Can you work these out from the model? Positions are in its coordinate system, mm. A direction names the side the tool comes from. Give positions to 0.01 mm unless a question says otherwise; leave off trailing zeros. Loops run counter-clockwise (first coordinate to the right, second up) from the corner with the lowest first, then second, coordinate; pieces in that order, holes last. Notation, with made-up numbers: (36, 62) -> (78, 62) arc R12 cw to (78, 71) -> close; hole circle Ø1 at (-9, 11). An arc over 180 degrees is marked (long way). Use CSV: the item, a comma, the result in double quotes.
Autodesk Inventor part; units mm, degrees
ref_plane "YZ Plane" through (0, 0, 0) normal (1, 0, 0) x (0, 1, 0)
ref_plane "XZ Plane" through (0, 0, 0) normal (0, 1, 0) x (-1, 0, 0)
ref_plane "XY Plane" through (0, 0, 0) normal (0, 0, 1) x (1, 0, 0)
sketch "Эскиз1" plane through (0, 0, 0) normal (0, 1, 0) x (-1, 0, 0)
  line L0 (0, 0) -> (8, 0) construction
  line L1 (8, 0) -> (8, 4)
  line L2 (8, 4) -> (13, 4)
  line L3 (13, 4) -> (13, 27)
  line L4 (13, 27) -> (20, 27)
  line L5 (0, 0) -> (0, 86)
  line L6 (0, 0) -> (-8, 0) construction
  line L7 (-8, 0) -> (-8, 4)
  line L8 (-8, 4) -> (-13, 4)
  line L9 (-13, 4) -> (-13, 27)
  line L10 (-13, 27) -> (-20, 27)
  line L11 (20, 27) -> (20, 44.5)
  line L12 (20, 44.5) -> (24, 44.5)
  line L13 (24, 44.5) -> (24, 64.5)
  line L14 (24, 64.5) -> (20, 64.5)
  line L15 (-20, 27) -> (-20, 44.5)
  line L16 (-20, 44.5) -> (-24, 44.5)
  line L17 (-24, 44.5) -> (-24, 64.5)
  line L18 (-24, 64.5) -> (-20, 64.5)
  line L19 (20, 64.5) -> (20, 82)
  line L20 (20, 82) -> (10, 82)
  line L21 (10, 82) -> (10, 86)
  line L22 (10, 86) -> (0, 86)
  line L23 (-20, 64.5) -> (-20, 82)
  line L24 (-20, 82) -> (-10, 82)
  line L25 (-10, 82) -> (-10, 86)
  line L26 (-10, 86) -> (0, 86)
  line L27 (-8, 0) -> (-8, -6)
  line L28 (8, -6) -> (8, 0)
  arc A0 (-8, -6) -> (8, -6) centre (0, -6) ccw
  circle A1 centre (0, -6) radius 5
  dimension "d0" = 16
  dimension "d1" = 26
  dimension "d2" = 40
  dimension "d3" = 4
  dimension "d4" = 23
  dimension "d5" = 55
  dimension "d6" = 20
  dimension "d7" = 20
  dimension "d10" = 6
  dimension "d11" = 10
extrude "Выдавливание1" add sketch "Эскиз1" along normal blind 4
properties part number "PistonPart3" material "Дерево (вишня)"
(1) If we section it at C-C, the plane z = 19: Write out the boundary of the cut face in (x, y), then the cut area to 3 significant figures.
Answer sheet:
outline,"(-13, 0) -> (13, 0) -> (13, 4) -> (-13, 4) -> close"
area,"104 mm2"
(2) If we section it at B-B, the plane x = 0: Write out the boundary of the cut face in (y, z).
Answer sheet:
outline,"(0, -14) -> (4, -14) -> (4, -11) -> (0, -11) -> close; (0, -1) -> (4, -1) -> (4, 86) -> (0, 86) -> close"
(3) Which directions (+Z, -Z, +X, -X, +Y, -Y) give clear straight access to the entire face, cutting with the end or side of a thin tool? Please do faces 1 (the face through (10, 2, 84)), 2 (the face through (13, 2, 15)), 3 (the face through (0, 4, 48)), 4 (the face through (-13, 2, 15)), 5 (the face through (-15, 2, 82)).
Answer sheet:
face 1,"+Z, +X, +Y, -Y"
face 2,"-Z, +X, +Y, -Y"
face 3,"+Z, -Z, +X, -X, +Y"
face 4,"-Z, -X, +Y, -Y"
face 5,"+Z, -X, +Y, -Y"
(4) If I drill on L1, parallel to Z at x = 0, y = 2.85; L2, parallel to Z at x = -21, y = 2.8; L3, parallel to Z at x = -16, y = 2.8, over which ranges is the centre line in solid material (lowest first)? Write a range as from..to.
Answer sheet:
L1,"z = -14..-11, -1..86"
L2,"z = 44.5..64.5"
L3,"z = 27..82"
(5) If we section it at A-A, the plane y = 2.3: Write out the boundary of the cut face in (x, z), then the cut area to 3 significant figures.
Answer sheet:
outline,"(-24, 44.5) -> (-20, 44.5) -> (-20, 27) -> (-13, 27) -> (-13, 4) -> (-8, 4) -> (-8, -6) arc R8 ccw to (8, -6) -> (8, 4) -> (13, 4) -> (13, 27) -> (20, 27) -> (20, 44.5) -> (24, 44.5) -> (24, 64.5) -> (20, 64.5) -> (20, 82) -> (10, 82) -> (10, 86) -> (-10, 86) -> (-10, 82) -> (-20, 82) -> (-20, 64.5) -> (-24, 64.5) -> close; hole circle Ø10 at (0, -6)"
area,"3,220 mm2"
(6) If we section it at D-D, the plane x = -16: Write out the boundary of the cut face in (y, z), then the cut area to 3 significant figures.
Answer sheet:
outline,"(0, 27) -> (4, 27) -> (4, 82) -> (0, 82) -> close"
area,"220 mm2"
(7) Will these pins go through, and if not, where does the flat tip stop? pin 1 Ø1 at (x, y) = (-2, 1) entering from -Z; pin 2 Ø1.5 at (x, y) = (-19, 1) entering from -Z; pin 3 Ø1.2 at (y, z) = (2, -3) entering from -X.
Answer sheet:
pin 1,"stops at z = -13.86"
pin 2,"stops at z = 27"
pin 3,"stops at x = -8"
